```python
from build123d import *

# Parameters (mm, degrees)
SKETCH1_R           = 25
BOSS_EXTRUDE1_DEPTH = 10
SKETCH2_W           = 50
SKETCH2_H           = 50
BOSS_EXTRUDE2_DEPTH = 0.1


with BuildPart() as part:
    # Sketch1 → Boss-Extrude1 (new body)
    with BuildSketch(Plane.XY):
        Polygon((0, 0), (0, 150), (60, 150), (60, 60), (150, 60), (150, 0), align=None)
        with Locations((30, 30)):
            Circle(SKETCH1_R, mode=Mode.SUBTRACT)
    extrude(amount=BOSS_EXTRUDE1_DEPTH)

    # Sketch2 → Boss-Extrude2 (add)
    with BuildSketch(Plane.XY.offset(10)):
        with Locations((30, 120)):
            Rectangle(SKETCH2_W, SKETCH2_H)
        with Locations((120, 30)):
            Rectangle(SKETCH2_W, SKETCH2_H)
    extrude(amount=BOSS_EXTRUDE2_DEPTH)


solid = part.part
```
Design review of the part built by this model. Coordinates are the model's own, in mm. A direction names the side the tool comes from. Give positions to 0.01 mm unless a question says otherwise; leave off trailing zeros. Loops run counter-clockwise (first coordinate to the right, second up) from the corner with the lowest first, then second, coordinate; pieces in that order, holes last. Notation, with made-up numbers: (-25.75, 66.25) -> (17.25, 66.25) arc R19 ccw to (17.25, 94.25) -> close; hole circle Ø4 at (-34.5, 11). An arc over 180 degrees is marked (long way). Write each question's results on one line, items separated by ' | '.
Q1. Take a section at D-D, the plane y = 115.5. Write out the cut boundary in (x, z), plus the area to 3 significant figures.
Reply:
outline: (0, 0) -> (60, 0) -> (60, 10) -> (55, 10) -> (55, 10.1) -> (5, 10.1) -> (5, 10) -> (0, 10) -> close | area: 605 mm²
Q2. The part is to be moulded in two halves that separate along X. For faces 1 (the face through (10, 15, 5)), 2 (the face through (150, 30, 5)), 3 (the face through (59, 59, 10)), say which applies: +X half, -X half, draft (parallel to the pull), parting line (faces both ways), or undercut.
Reply:
face 1: undercut | face 2: +X half | face 3: draft
Q3. Take a section at A-A, the plane z = 2.5. Write out the cut boundary in (x, y).
Reply:
outline: (0, 0) -> (150, 0) -> (150, 60) -> (60, 60) -> (60, 150) -> (0, 150) -> close; hole circle Ø50 at (30, 30)
Q4. Wall thickness on L1, parallel to Y at x = 30, z = 3; L2, parallel to Y at x = 70, z = 3.5: over which ranges is each line inside the solid? List them lowest first.
Reply:
L1: y = 0 to 5, 55 to 150 | L2: y = 0 to 60
Q5. Take a section at B-B, the plane x = 30. Write out the cut boundary in (y, z).
Reply:
outline: (0, 0) -> (5, 0) -> (5, 10) -> (0, 10) -> close; (55, 0) -> (150, 0) -> (150, 10) -> (145, 10) -> (145, 10.1) -> (95, 10.1) -> (95, 10) -> (55, 10) -> close
Q6. Take a section at C-C, the plane y = 38.5. Write out the cut boundary in (x, z), plus the area to 3 significant figures.
Reply:
outline: (0, 0) -> (6.49, 0) -> (6.49, 10) -> (0, 10) -> close; (53.51, 0) -> (150, 0) -> (150, 10) -> (145, 10) -> (145, 10.1) -> (95, 10.1) -> (95, 10) -> (53.51, 10) -> close | area: 1,030 mm²
Q7. For pin 1 Ø2 at (x, z) = (96, 7) entering from +Y; pin 2 Ø1 at (y, z) = (61.5, 7) entering from +X, all flat-tipped, find the tip position at first contact; note any pin that passes through.
Reply:
pin 1: stops at y = 60 | pin 2: stops at x = 60
Q8. Machinability: for faces 4 (the face through (104, 60, 5)), 5 (the face through (30, 150, 5)), which of the approach directions +Z, -Z, +X, -X, +Y, -Y give a long, thin tool a straight path to every point of the face, cutting with its end or side? Answer none if there is none.
Reply:
face 4: +Z, -Z, +X, +Y | face 5: +Z, -Z, +X, -X, +Y
